Could you check a few things on this model? Use its own coordinates, in mm. A direction names the side the tool comes from. Round coordinates to 2 decimals unless told otherwise and drop trailing zeros. Loops run counter-clockwise (first coordinate to the right, second up) from the corner with the lowest first, then second, coordinate; pieces in that order, holes last. Notation, with made-up numbers: M 18,32.25 L 47,32.25 A24 ccw 47,47.25 Z; hole C -6,20 d10. An arc over 180 degrees is marked long. One line per item, written item: value. Start each with the question number.
Q1. Thinking about a two-plate mould opening in Z: for faces 1 (the face through (0, 5, 43.18)), 2 (the face through (1.651, 7, 6)), 3 (the face through (0, 1, 0)), which applies, released by +Z, released by -Z, zero draft, split by the parting line, or undercut?
Q2. I'm going to push flat-ended pins straight in: pin 1 Ø1.8 at (y, z) = (7, 4.5) entering from -X; pin 2 Ø2 at (x, z) = (4.5, 38) entering from +Y; pin 3 Ø5 at (y, z) = (-2, 34.5) entering from +X. Where does each tip first touch, or does it pass through?
Q3. Imagine slicing it at D-D (z = 30.5). Please give me the cut outline in (x, y).
Q4. Imagine slicing it at A-A (x = 0). Please give me the cut outline in (y, z), then the cut area to 3 significant figures.
Q5. Which directions (+Z, -Z, +X, -X, +Y, -Y) give clear straight access to the entire face, cutting with the end or side of a thin tool? Please do faces 4 (the face through (1.143, 5, 50)), 5 (the face through (0, 5.832, 50)), 6 (the face through (-1.651, 7, 6)).
Q6. Please list where these lines run through material, in increasing order: line 1 along Z through (x, y) = (3.75, -3.5); line 2 along Z through (x, y) = (0.25, 6.25); line 3 along X through (y, z) = (5.75, 51).
Q7. Imagine slicing it at C-C (y = -4.25). Please give me the cut outline in (x, z), then the cut area to 3 significant figures.
Q8. Imagine slicing it at B-B (z = 10). Please give me the cut outline in (x, y), then the cut area to 3 significant figures.
from build123d import *

# Parameters (mm, degrees)
SKETCH1_R                = 6.223
BOSS_EXTRUDE1_DEPTH      = 28.194
SKETCH2_R                = 4.826
BOSS_EXTRUDE2_DEPTH      = 27.686
BOSS_EXTRUDE2_DEPTH_BACK = 5.08
SKETCH3_W                = 2.286
SKETCH3_H                = 2.286
BOSS_EXTRUDE3_DEPTH      = 12.7
SKETCH4_W                = 3.302
SKETCH4_H                = 3.302
BOSS_EXTRUDE4_DEPTH      = 12.7


with BuildPart() as part:
    # Sketch1 → Boss-Extrude1 (new body)
    with BuildSketch(Plane.XY):
        Circle(SKETCH1_R)
    extrude(amount=BOSS_EXTRUDE1_DEPTH)

    # Sketch2 → Boss-Extrude2 (add, two sides)
    with BuildSketch(Plane.XY.offset(28.194)) as boss_extrude2_sk:
        Circle(SKETCH2_R)
    extrude(amount=BOSS_EXTRUDE2_DEPTH)
    extrude(boss_extrude2_sk.sketch, amount=-BOSS_EXTRUDE2_DEPTH_BACK)

    # Sketch3 → Boss-Extrude3 (add)
    with BuildSketch(Plane.XY.offset(55.88)):
        with Locations((0, 4.688691395)):
            Rectangle(SKETCH3_W, SKETCH3_H)
    extrude(amount=-BOSS_EXTRUDE3_DEPTH)

    # Sketch4 → Boss-Extrude4 (add)
    with BuildSketch(Plane(origin=(0, 0, 0), x_dir=(-1, 0, 0), z_dir=(0, 0, -1))):
        with Locations((0, 5.999994)):
            Rectangle(SKETCH4_W, SKETCH4_H)
    extrude(amount=-BOSS_EXTRUDE4_DEPTH)


solid = part.part
Report:
1. face 1: undercut
1. face 2: zero draft
1. face 3: released by -Z
2. pin 1: stops at x = -1.65
2. pin 2: stops at y = 3.32
2. pin 3: stops at x = 4.83
3. outline: C 0,0 d9.65
4. outline: M -6.22,0 L 7.65,0 L 7.65,12.7 L 6.22,12.7 L 6.22,28.19 L 4.83,28.19 L 4.83,43.18 L 5.83,43.18 L 5.83,55.88 L -4.83,55.88 L -4.83,28.19 L -6.22,28.19 Z
4. area: 649 mm²
5. face 4: +Z, +X, +Y
5. face 5: +Z, +X, -X, +Y
5. face 6: +Z, -Z, -X, +Y
6. line 1: z = 0 to 28.19
6. line 2: z = 0 to 12.7
6. line 3: x = -1.14 to 1.14
7. outline: M -4.55,0 L 4.55,0 L 4.55,28.19 L 2.29,28.19 L 2.29,55.88 L -2.29,55.88 L -2.29,28.19 L -4.55,28.19 Z
7. area: 383 mm²
8. outline: M -1.65,6 A6.22 ccw long 1.65,6 L 1.65,7.65 L -1.65,7.65 Z
8. area: 127 mm²
